Drawing for the job (mm, zero at the part's lowest x, y, z). A direction names the side the tool comes from. Coordinates: 2 decimals unless noted, no trailing zeros. Loops run counter-clockwise (first coordinate to the right, second up) from the corner with the lowest first, then second, coordinate; pieces in that order, holes last. Notation, with made-up numbers: (-29, 54.25) - (-16, 54.25) arc R34 cw to (-16, 90.25) - close; hole circle Ø5 at (59.25, -3.5). An arc over 180 degrees is marked (long way). One line per item, written item: value.
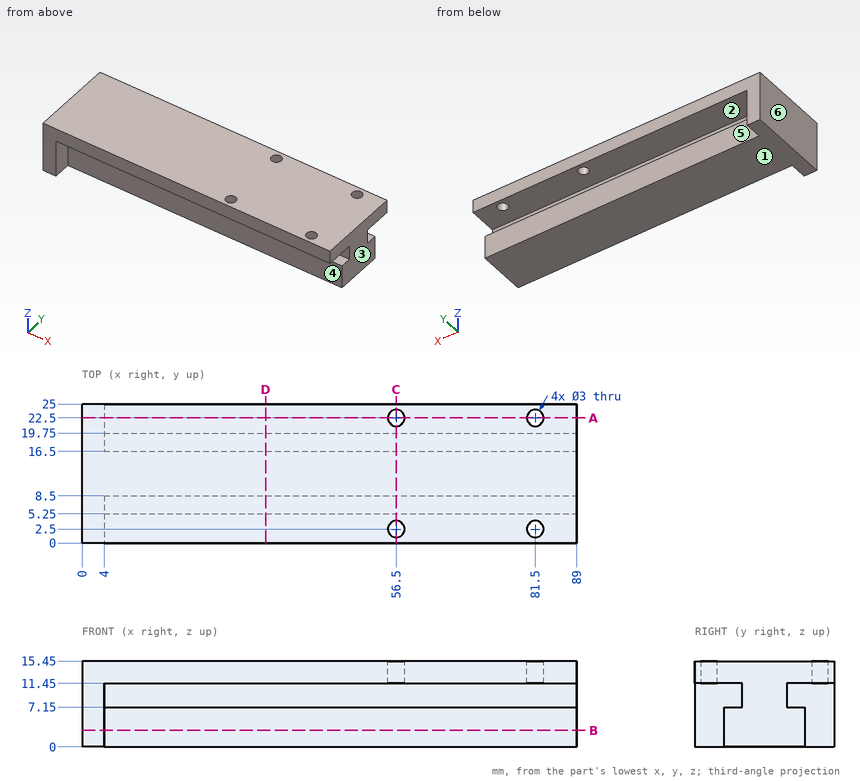
Item 1: Pull direction Z, two halves, no side cores. Call the marked faces 1, 2 and 3: released by +Z, released by -Z, zero draft, split by the parting line, or undercut.
Check result:
face 1: released by -Z
face 2: undercut
face 3: zero draft
Item 2: Drop flat-ended pins along their axis: P1, Ø4, axis at x = 81.5, y = 22.5, coming from the -Z side; P2, Ø2, axis at x = 57.5, z = 3, coming from the +Y side; P3, Ø8, axis at x = 40, z = 2, coming from the -Y side. Give the stop position or say it passes through.
Check result:
P1: stops at z = 11.45
P2: stops at y = 19.75
P3: stops at y = 5.25
Item 3: Cut at D-D, the plane x = 33. Write the cut outline in (y, z), then the cut area to 3 significant figures.
Check result:
outline: (0, 11.45) - (8.5, 11.45) - (8.5, 7.15) - (5.25, 7.15) - (5.25, 0) - (19.75, 0) - (19.75, 7.15) - (16.5, 7.15) - (16.5, 11.45) - (25, 11.45) - (25, 15.45) - (0, 15.45) - close
area: 238 mm^2
Item 4: Probe probe 1 along X at (y, z) = (2.5, 13.95); probe 2 along Y at (x, z) = (56.5, 14.55); probe 3 along Z at (x, y) = (25.5, 17.5). List the from-to ranges inside material, lowest first. Write a range as from..to.
Check result:
probe 1: x = 0..55, 58..80, 83..89
probe 2: y = 0..1, 4..21, 24..25
probe 3: z = 0..7.15, 11.45..15.45
Item 5: Tool access for the marked faces 4, 5 and 6: list every direction of +Z, -Z, +X, -X, +Y, -Y with a clear straight run to the whole face (end or side of a thin tool).
Check result:
face 4: -Z, +X, -Y
face 5: -Z, +X, +Y
face 6: +Z, -Z, -X, +Y, -Y
Item 6: Cut at B-B, the plane z = 3. Write the cut outline in (x, y).
Check result:
outline: (0, 0) - (4, 0) - (4, 5.25) - (89, 5.25) - (89, 19.75) - (4, 19.75) - (4, 25) - (0, 25) - close
Item 7: Cut at C-C, the plane x = 56.5. Write the cut outline in (y, z), then the cut area to 3 significant figures.
Check result:
outline: (0, 11.45) - (1, 11.45) - (1, 15.45) - (0, 15.45) - close; (4, 11.45) - (8.5, 11.45) - (8.5, 7.15) - (5.25, 7.15) - (5.25, 0) - (19.75, 0) - (19.75, 7.15) - (16.5, 7.15) - (16.5, 11.45) - (21, 11.45) - (21, 15.45) - (4, 15.45) - close; (24, 11.45) - (25, 11.45) - (25, 15.45) - (24, 15.45) - close
area: 214 mm^2
Item 8: Cut at A-A, the plane y = 22.5. Write the cut outline in (x, z), then the cut area to 3 significant figures.
Check result:
outline: (0, 0) - (4, 0) - (4, 11.45) - (55, 11.45) - (55, 15.45) - (0, 15.45) - close; (58, 11.45) - (80, 11.45) - (80, 15.45) - (58, 15.45) - close; (83, 11.45) - (89, 11.45) - (89, 15.45) - (83, 15.45) - close
area: 378 mm^2
